The model under review builds one solid part; all positions refer to its coordinate system, in mm. A direction names the side the tool comes from. Give positions to 0.01 mm unless a question says otherwise; leave off trailing zeros. Loops run counter-clockwise (first coordinate to the right, second up) from the corner with the lowest first, then second, coordinate; pieces in that order, holes last. Notation, with made-up numbers: (-31, 1.25) -> (10, 1.25) arc R25 cw to (10, 39.25) -> close; hole circle Ø11 at (23.5, 1). An arc over 180 degrees is marked (long way). Write each question's results on one line, items separated by ' | '. Start each with the question number.
Q1. Wall thickness on L1, parallel to X at y = 0, z = -3.35; L2, parallel to X at y = -15.5, z = 6.3; L3, parallel to Y at x = -15.5, z = 8.45: over which ranges is each line inside the solid? List them lowest first. Write a range as [from, to].
Q2. Machinability: for faces 1 (the face through (-19, 19, 7)), 2 (the face through (-15.923, -18.722, 6.232)), 3 (the face through (8, -1.47, 3.94)), which of the approach directions +Z, -Z, +X, -X, +Y, -Y give a long, thin tool a straight path to every point of the face, cutting with its end or side? Answer none if there is none.
Q3. We need section C-C (z = 3). Write out the cut boundary in (x, y), plus the area to 3 significant figures.
Q4. Insertion check: pin 1 Ø8 at (x, z) = (10.5, 2.5) entering from -Y; pin 2 Ø5 at (x, y) = (-14, 16) entering from -Z; pin 3 Ø6 at (x, z) = (-14, -0.5) entering from +Y; pin 4 Ø1.7 at (x, y) = (-10.5, 0.5) entering from +Z. Each pin has a flat end and moves straight along its axis. Give the tip position at first contact, or say it passes through.
Q5. We need section B-B (y = 15.5). Write out the cut boundary in (x, z).
Q6. Mouldability with a two-part tool opening along Y and no side actions: class faces 4 (the face through (-14.985, -0.66, 0.07)), 5 (the face through (-12.1, -0.07, -2.46)), 6 (the face through (-4, -4, -5)) as released by +Y, released by -Y, zero draft, split by the parting line, or undercut.
Q7. We need section A-A (x = 0). Write out the cut boundary in (y, z).
from build123d import *

# Parameters (mm, degrees)
F0_R      = 15
F0_R_2    = 1.6
F0_R_3    = 5
F1_DEPTH  = 5
F2_W      = 42
F2_H      = 42
F2_R      = 1.6
F2_R_2    = 15
F2_R_3    = 5
F3_DEPTH  = 5
F4_SIZE   = 4
F5_R      = 5
F6_DEPTH  = 2
F7_R      = 15
F7_R_2    = 1.6
F7_R_3    = 5
F8_DEPTH  = 5
F9_R      = 1.6
F10_DEPTH = 5
F11_R     = 3.25
F11_R_2   = 1.6
F12_DEPTH = 2.5


with BuildPart() as f1:
    # F0 (on Top) → F1 (new body)
    with BuildSketch(Plane.XY):
        Circle(F0_R)
        with Locations((-10.5, 0)):
            Circle(F0_R_2, mode=Mode.SUBTRACT)
        Circle(F0_R_3, mode=Mode.SUBTRACT)
        with Locations((10.5, 0)):
            Circle(F0_R_2, mode=Mode.SUBTRACT)
    extrude(amount=F1_DEPTH)

    # F2 (on face) → F3 (join)
    with BuildSketch(Plane.XY.offset(5)):
        Rectangle(F2_W, F2_H)
        with Locations((-15.5, -15.5)):
            Circle(F2_R, mode=Mode.SUBTRACT)
        with Locations((15.5, -15.5)):
            Circle(F2_R, mode=Mode.SUBTRACT)
        with Locations((-15.5, 15.5)):
            Circle(F2_R, mode=Mode.SUBTRACT)
        Circle(F2_R_2, mode=Mode.SUBTRACT)
        with Locations((15.5, 15.5)):
            Circle(F2_R, mode=Mode.SUBTRACT)
        Circle(F2_R_2)
        Polygon((-13.8486315613, 0), (-12.1743157806, 2.9), (-8.8256842194, 2.9), (-7.1513684387, 0), (-8.8256842194, -2.9), (-12.1743157806, -2.9), align=None, mode=Mode.SUBTRACT)
        Circle(F2_R_3, mode=Mode.SUBTRACT)
        Polygon((13.8486315613, 0), (12.1743157806, -2.9), (8.8256842194, -2.9), (7.1513684387, 0), (8.8256842194, 2.9), (12.1743157806, 2.9), align=None, mode=Mode.SUBTRACT)
    extrude(amount=F3_DEPTH)

    # F4
    f4_edges = [f1.edges().sort_by_distance(p)[0] for p in [
        (21, 21, 7.5),
        (21, -21, 7.5),
        (-21, -21, 7.5),
        (-21, 21, 7.5),
    ]]
    chamfer(f4_edges, length=F4_SIZE)

    # F5 (on face) → F6 (cut)
    with BuildSketch(Plane.XY.offset(10)):
        with BuildLine():
            Line((8.8256842194, 2.9), (10.6108435103, 2.9))
            ThreePointArc((10.6108435103, 2.9), (0, 11), (-10.6108435103, 2.9))
            Line((-10.6108435103, 2.9), (-8.8256842194, 2.9))
            Line((-8.8256842194, 2.9), (-7.1513684387, 0))
            Line((-7.1513684387, 0), (-8.8256842194, -2.9))
            Line((-8.8256842194, -2.9), (-10.6108435103, -2.9))
            ThreePointArc((-10.6108435103, -2.9), (0, -11), (10.6108435103, -2.9))
            Line((10.6108435103, -2.9), (8.8256842194, -2.9))
            Line((8.8256842194, -2.9), (7.1513684387, 0))
            Line((7.1513684387, 0), (8.8256842194, 2.9))
        make_face()
        Circle(F5_R, mode=Mode.SUBTRACT)
    extrude(amount=-F6_DEPTH, mode=Mode.SUBTRACT)

    # F7 (on face) → F8 (join)
    with BuildSketch(Plane(origin=(0, 0, 0), x_dir=(1, 0, 0), z_dir=(0, 0, -1))):
        Circle(F7_R)
        with Locations((-10.5, 0)):
            Circle(F7_R_2, mode=Mode.SUBTRACT)
        Circle(F7_R_3, mode=Mode.SUBTRACT)
        with Locations((10.5, 0)):
            Circle(F7_R_2, mode=Mode.SUBTRACT)
    extrude(amount=F8_DEPTH)

    # F9 (on face) → F10 (cut)
    with BuildSketch(Plane.XY.offset(5)):
        Polygon((-12.1743157806, 2.9), (-13.8486315613, 0), (-12.1743157806, -2.9), (-8.8256842194, -2.9), (-7.1513684387, 0), (-8.8256842194, 2.9), align=None)
        with Locations((-10.5, 0)):
            Circle(F9_R, mode=Mode.SUBTRACT)
        Polygon((8.8256842194, -2.9), (12.1743157806, -2.9), (13.8486315613, 0), (12.1743157806, 2.9), (8.8256842194, 2.9), (7.1513684387, 0), align=None)
    extrude(amount=-F10_DEPTH, mode=Mode.SUBTRACT)

    # F11 (on face) → F12 (cut)
    with BuildSketch(Plane(origin=(0, 0, 5), x_dir=(1, 0, 0), z_dir=(0, 0, -1))):
        with Locations((15.5, 15.5)):
            Circle(F11_R)
        with Locations((15.5, 15.5)):
            Circle(F11_R_2, mode=Mode.SUBTRACT)
        with Locations((15.5, -15.5)):
            Circle(F11_R)
        with Locations((15.5, -15.5)):
            Circle(F11_R_2, mode=Mode.SUBTRACT)
        with Locations((-15.5, -15.5)):
            Circle(F11_R)
        with Locations((-15.5, -15.5)):
            Circle(F11_R_2, mode=Mode.SUBTRACT)
        with Locations((-15.5, 15.5)):
            Circle(F11_R)
        with Locations((-15.5, 15.5)):
            Circle(F11_R_2, mode=Mode.SUBTRACT)
    extrude(amount=-F12_DEPTH, mode=Mode.SUBTRACT)


solid = f1.part
Output:
1) L1: [-15, -12.1], [-8.9, -5], [5, 8.9], [12.1, 15] | L2: [-21, -18.75], [-12.25, 12.25], [18.75, 21] | L3: [-21, -17.1], [-13.9, 13.9], [17.1, 21]
2) face 1: +Z, -Z, -X, +Y | face 2: -Z | face 3: +Z
3) outline: circle Ø30 at (0, 0); hole (-13.85, 0) -> (-12.17, -2.9) -> (-8.83, -2.9) -> (-7.15, 0) -> (-8.83, 2.9) -> (-12.17, 2.9) -> close; hole circle Ø10 at (0, 0); hole (7.15, 0) -> (8.83, -2.9) -> (12.17, -2.9) -> (13.85, 0) -> (12.17, 2.9) -> (8.83, 2.9) -> close | area: 570 mm2
4) pin 1: y = -21 | pin 2: z = 5 | pin 3: y = 10.2 | pin 4: through
5) outline: (-21, 5) -> (-18.75, 5) -> (-18.75, 7.5) -> (-17.1, 7.5) -> (-17.1, 10) -> (-21, 10) -> close; (-13.9, 7.5) -> (-12.25, 7.5) -> (-12.25, 5) -> (12.25, 5) -> (12.25, 7.5) -> (13.9, 7.5) -> (13.9, 10) -> (-13.9, 10) -> close; (17.1, 7.5) -> (18.75, 7.5) -> (18.75, 5) -> (21, 5) -> (21, 10) -> (17.1, 10) -> close
6) face 4: split by the parting line | face 5: undercut | face 6: zero draft
7) outline: (-21, 5) -> (-15, 5) -> (-15, -5) -> (-5, -5) -> (-5, 8) -> (-11, 8) -> (-11, 10) -> (-21, 10) -> close; (5, -5) -> (15, -5) -> (15, 5) -> (21, 5) -> (21, 10) -> (11, 10) -> (11, 8) -> (5, 8) -> close
